```python
from build123d import *

# Parameters (mm, degrees)
SKETCH1_R                  = 4.7625
BOSS_EXTRUDE1_DEPTH        = 13.335
SKETCH2_R                  = 2
CUT_EXTRUDE1_DEPTH         = 28.507302894
F_4_40_TAPPED_HOLE1_REACH  = 19.065
F_4_40_TAPPED_HOLE1_BORE_R = 1.1303
CUT_EXTRUDE2_DEPTH         = 1.190625
CHAMFER1_SIZE              = 0.254


with BuildPart() as part:
    # Sketch1 → Boss-Extrude1 (new, symmetric)
    with BuildSketch(Plane(origin=(0, 0, 0), x_dir=(0, 0, -1), z_dir=(1, 0, 0))):
        Circle(SKETCH1_R)
    extrude(amount=BOSS_EXTRUDE1_DEPTH, both=True)

    # Sketch2 → Cut-Extrude1 (cut, through all)
    with BuildSketch(Plane(origin=(13.335, 0, 0), x_dir=(0, 0, -1), z_dir=(1, 0, 0))):
        Circle(SKETCH2_R)
    extrude(amount=-CUT_EXTRUDE1_DEPTH, mode=Mode.SUBTRACT)

    # #4-40 Tapped Hole1 bore → #4-40 Tapped Hole1 (cut, up to next)
    with BuildSketch(Plane.XY.offset(4.7625), mode=Mode.PRIVATE) as f_4_40_tapped_hole1_sk1:
        with Locations((-9.017, 0)):
            Circle(F_4_40_TAPPED_HOLE1_BORE_R)
    f_4_40_tapped_hole1_tool1 = extrude(f_4_40_tapped_hole1_sk1.sketch, amount=-F_4_40_TAPPED_HOLE1_REACH, mode=Mode.PRIVATE) & part.part
    # #4-40 Tapped Hole1 bore → #4-40 Tapped Hole1 (cut, up to next)
    with BuildSketch(Plane.XY.offset(4.7625), mode=Mode.PRIVATE) as f_4_40_tapped_hole1_sk2:
        with Locations((-3.937, 0)):
            Circle(F_4_40_TAPPED_HOLE1_BORE_R)
    f_4_40_tapped_hole1_tool2 = extrude(f_4_40_tapped_hole1_sk2.sketch, amount=-F_4_40_TAPPED_HOLE1_REACH, mode=Mode.PRIVATE) & part.part
    add(f_4_40_tapped_hole1_tool1.solids().sort_by_distance((-9.017, 0, 4.7625))[0], mode=Mode.SUBTRACT)
    add(f_4_40_tapped_hole1_tool2.solids().sort_by_distance((-3.937, 0, 4.7625))[0], mode=Mode.SUBTRACT)

    # Sketch7 → Cut-Extrude2 (cut)
    with BuildSketch(Plane(origin=(0, 0, -4.7625), x_dir=(-1, 0, 0), z_dir=(0, 0, -1))):
        with BuildLine():
            Line((-4.7625, 1.190625), (7.9375, 1.190625))
            ThreePointArc((7.9375, 1.190625), (9.128125, 0), (7.9375, -1.190625))
            Line((7.9375, -1.190625), (-4.7625, -1.190625))
            ThreePointArc((-4.7625, -1.190625), (-5.953125, 0), (-4.7625, 1.190625))
        make_face()
    extrude(amount=-CUT_EXTRUDE2_DEPTH, mode=Mode.SUBTRACT)

    # Chamfer1
    chamfer1_edges = [part.edges().sort_by_distance(p)[0] for p in [
        (-13.335, 0, 4.7625),
        (13.335, 0, 4.7625),
        (-13.335, 0, 2),
        (13.335, 0, 2),
    ]]
    chamfer(chamfer1_edges, length=CHAMFER1_SIZE)


solid = part.part
```
Can you work these out from the model? Positions are in its coordinate system, mm. A direction names the side the tool comes from. Give positions to 0.01 mm unless a question says otherwise; leave off trailing zeros. Loops run counter-clockwise (first coordinate to the right, second up) from the corner with the lowest first, then second, coordinate; pieces in that order, holes last. Notation, with made-up numbers: M 45,85 L 86,85 A15 cw 86,90 Z; hole C 80.25,75.5 d4. An arc over 180 degrees is marked long. Use CSV: the item, a comma, the result in double quotes. Start each with the question number.
1. If I drill on L1, parallel to Y at x = 0, z = 0; L2, parallel to Z at x = 5, y = 0; L3, parallel to Z at x = 1, y = 1.75, over which ranges is the centre line in solid material (lowest first)?
2. Imagine slicing it at C-C, the plane x = -0.25. Write out the boundary of the cut face in (y, z) (1 decimal).
3. Imagine slicing it at D-D, the plane x = 10.5. Write out the boundary of the cut face in (y, z) (1 decimal).
4. For P1, Ø1.5, axis at x = -4.5, z = 2.5, coming from the -Y side; P2, Ø1.5, axis at x = 9, z = -3, coming from the +Y side; P3, Ø1.9, axis at x = -1.5, y = -0.5, coming from the -Z side, each with a flat end and sliding along its axis, tell me the tip position at first contact or that it passes through.
5. If we mould it in two halves opening along Z, with no side actions, what happens to faces 1 (the face through (-2, 0, -3.572)), 2 (the face through (0.183, -0.766, -1.847)), 3 (the face through (-13.335, -2, -2))? For each: released by +Z, released by -Z, zero draft, split by the parting line, or undercut.
6. On a 3-axis mill with a long thin cutter (end or side, diameter ignored), from which of +Z, -Z, +X, -X, +Y, -Y can I reach the whole of each face in a straight line? I mean faces 4 (the face through (-2.89, -0.43, 3.23)), 5 (the face through (13.335, -2, -2)), 6 (the face through (-9.128, 0.026, -4.176)). Say none if no direction works.
7. Imagine slicing it at B-B, the plane y = 0. Count the separate pieces of the cut face and the enclosed holes in it, plus the area to 3 significant figures.
Response values:
1,L1,"-4.76 to -2, 2 to 4.76"
1,L2,"-3.57 to -2, 2 to 4.76"
1,L3,"-4.43 to -0.97, 0.97 to 4.43"
2,outline,"M -1.2,-4.6 L -1.2,-3.6 L 1.2,-3.6 L 1.2,-4.6 A4.8 ccw long Z; hole C 0,0 d4"
3,outline,"C 0,0 d9.5; hole C 0,0 d4"
4,P1,"y = -4.43"
4,P2,"y = 4.2"
4,P3,"z = -4.61"
5,face 1,"released by -Z"
5,face 2,"undercut"
5,face 3,"zero draft"
6,face 4,"+Z"
6,face 5,"+Z, -Z, +X, +Y, -Y"
6,face 6,"-Z"
7,separate pieces,"4"
7,enclosed holes,"0"
7,area,"117 mm^2"
